The model under review builds one solid part; all positions refer to its coordinate system, in mm. Face numbers are marked on the shaded views. Round coordinates to 2 decimals unless told otherwise and drop trailing zeros. Order: outer loops, then holes, each group sorted by start corner. A loop starts at its lowest first (then second) coordinate and runs counter-clockwise, first axis right, second up. Notation, with made-up numbers: M -22.5,52 L -18.5,52 A25 ccw -18.5,79 Z; hole C -32,38.25 d6. An arc over 180 degrees is marked long. Answer as a JSON object with one key per item and string values. Group by question number.
1) To check wall thickness, follow line 1 (Y direction, x = 0, z = -4.5); line 2 (Z direction, x = 1.5, y = 4.5); line 3 (X direction, y = -4.5, z = -1.25). State the ranges of each line that lie inside material, in increasing order.
2) The part is to be moulded in two halves that separate along X. For the marked faces 1 and 2, say which applies: +X half, -X half, draft (parallel to the pull), parting line (faces both ways), or undercut.
3) Insertion check: pin 1 Ø1 at (x, z) = (7, -1.5) entering from +Y; pin 2 Ø1.5 at (y, z) = (9.5, 1) entering from +X; pin 3 Ø4.5 at (x, y) = (-1, -11.5) entering from -Z. Each pin has a flat end and moves straight along its axis. Give the tip position at first contact, or say it passes through.
4) Consider section A-A, the plane z = -2. Write out the cut boundary in (x, y), then the cut area to 3 significant figures.
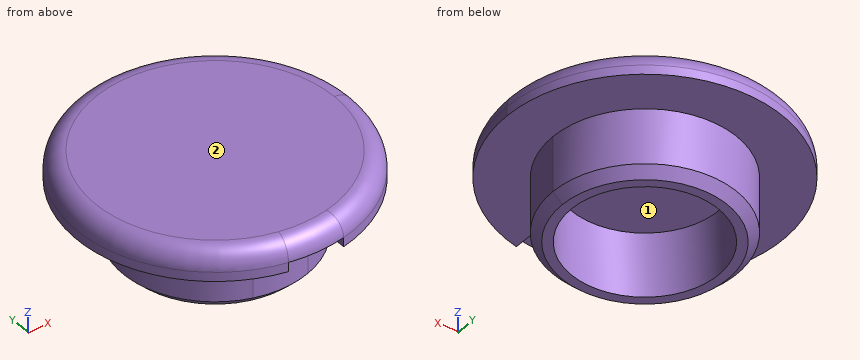
```python
from build123d import *
from build123d import SkipClean  # not in build123d's __all__

# Parameters (mm, degrees)
F0_R     = 8
F1_DEPTH = 3
F2_DEPTH = 7
F3_R     = 2
F4_SIZE  = 1
F5_DEPTH = 1


with BuildPart() as f1:
    # F0 (on Top) → F1 (new body)
    with BuildSketch(Plane.XY):
        with BuildLine():
            ThreePointArc((-3, -9.5393920142), (-5.9160797831, 8.0622577483), (10, 0))
            ThreePointArc((10, 0), (8.0622577483, -5.9160797831), (3, -9.5393920142))
            Line((3, -9.5393920142), (3, -14.6969384567))
            ThreePointArc((3, -14.6969384567), (11.6189500386, -9.4868329805), (15, 0))
            ThreePointArc((15, 0), (-9.4868329805, 11.6189500386), (-3, -14.6969384567))
            Line((-3, -14.6969384567), (-3, -9.5393920142))
        make_face()
        with BuildLine():
            ThreePointArc((3, -9.5393920142), (0, -10), (-3, -9.5393920142))
            Line((-3, -9.5393920142), (-3, -14.6969384567))
            ThreePointArc((-3, -14.6969384567), (0, -15), (3, -14.6969384567))
            Line((3, -14.6969384567), (3, -9.5393920142))
        make_face()
        with BuildLine():
            ThreePointArc((3, -9.5393920142), (8.0622577483, -5.9160797831), (10, 0))
            ThreePointArc((10, 0), (-5.9160797831, 8.0622577483), (-3, -9.5393920142))
            ThreePointArc((-3, -9.5393920142), (0, -10), (3, -9.5393920142))
        make_face()
        Circle(F0_R, mode=Mode.SUBTRACT)
        Circle(F0_R)
    extrude(amount=F1_DEPTH)

    # F0 (on Top) → F2 (join)
    with BuildSketch(Plane.XY):
        with BuildLine():
            ThreePointArc((3, -9.5393920142), (8.0622577483, -5.9160797831), (10, 0))
            ThreePointArc((10, 0), (-5.9160797831, 8.0622577483), (-3, -9.5393920142))
            ThreePointArc((-3, -9.5393920142), (0, -10), (3, -9.5393920142))
        make_face()
        Circle(F0_R, mode=Mode.SUBTRACT)
    extrude(amount=-F2_DEPTH)

    # F3
    f3_edges = [f1.edges().sort_by_distance(p)[0] for p in [
        (-15, 0, 3),
    ]]
    fillet(f3_edges, radius=F3_R)

    # F4
    f4_edges = [f1.edges().sort_by_distance(p)[0] for p in [
        (3, 9.539392, -7),
    ]]
    chamfer(f4_edges, length=F4_SIZE)

    # F0 (on Top) → F5 (cut)
    with BuildSketch(Plane.XY):
        with BuildLine():
            ThreePointArc((3, -9.5393920142), (0, -10), (-3, -9.5393920142))
            Line((-3, -9.5393920142), (-3, -14.6969384567))
            ThreePointArc((-3, -14.6969384567), (0, -15), (3, -14.6969384567))
            Line((3, -14.6969384567), (3, -9.5393920142))
        make_face()
    with SkipClean():  # cleaning this boolean's faces spoils the solid; the shape is the same uncleaned
        extrude(amount=F5_DEPTH, mode=Mode.SUBTRACT)


solid = f1.part
```
Results list:
{
 "1": {"line 1": "-10 to -8, 8 to 10", "line 2": "0 to 3", "line 3": "-8.93 to -6.61, 6.61 to 8.93"},
 "2": {"face 1": "undercut", "face 2": "draft"},
 "3": {"pin 1": "y = 7.6", "pin 2": "x = 12.18", "pin 3": "z = -6.71"},
 "4": {"outline": "C 0,0 d20; hole C 0,0 d16", "area": "113 mm^2"}
}
